Here's how the part is built. I have some questions about the finished solid (model axes, mm). Round coordinates to 2 decimals unless told otherwise and drop trailing zeros. Order: outer loops, then holes, each group sorted by start corner. A loop starts at its lowest first (then second) coordinate and runs counter-clockwise, first axis right, second up.
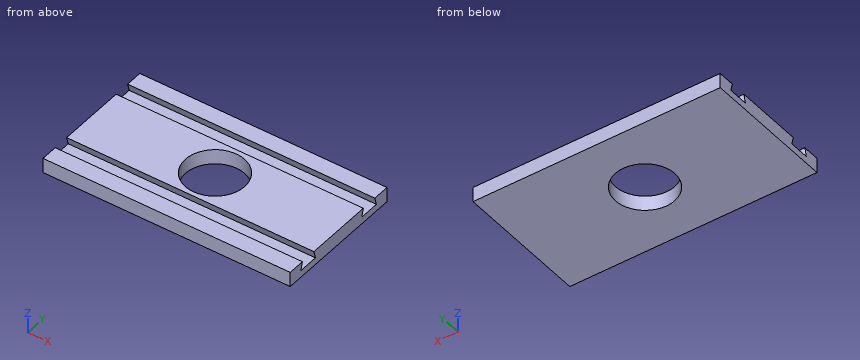
```python
from build123d import *

# Parameters (mm, degrees)
PLATE_PROFILE_W             = 100
PLATE_PROFILE_H             = 54
PLATE_PROFILE_R             = 12
PLATE_6MM_DEPTH             = 6
DOVETAIL_GROOVES_DEPTH      = 58.140178509
DOVETAIL_GROOVES_DEPTH_BACK = 58.140178509


with BuildPart() as part:
    # Plate profile → Plate 6mm (new body)
    with BuildSketch(Plane.XY):
        Rectangle(PLATE_PROFILE_W, PLATE_PROFILE_H)
        Circle(PLATE_PROFILE_R, mode=Mode.SUBTRACT)
    extrude(amount=-PLATE_6MM_DEPTH)

    # Groove profiles → Dovetail grooves (cut, two sides: drawn at the far end of the back side and taken through both)
    with BuildSketch(Plane(origin=(0, 0, 0), x_dir=(0, 0, -1), z_dir=(1, 0, 0)).offset(-DOVETAIL_GROOVES_DEPTH_BACK)):
        Polygon((-0.2, 13.846344337), (3.2, 12.939677671), (3.2, 21.060322329), (-0.2, 20.153655663), align=None)
        Polygon((-0.2, -13.846344337), (3.2, -12.939677671), (3.2, -21.060322329), (-0.2, -20.153655663), align=None)
    extrude(amount=DOVETAIL_GROOVES_DEPTH + DOVETAIL_GROOVES_DEPTH_BACK, mode=Mode.SUBTRACT)


solid = part.part
```
1) If we section it at A-A (y = 0): Write out the boundary of the cut face in (x, z), plus the area to 3 significant figures.
2) I'm going to push flat-ended pins straight in: pin 1 (6.5 mm diameter, centred on x = 9.5, y = -17, fed in from +Z); pin 2 (4 mm diameter, centred on x = 0, y = 16, fed in from +Z). Where does each tip first touch, or does it pass through?
3) If we section it at D-D (z = -4.7): Write out the boundary of the cut face in (x, y), plus the area to 3 significant figures.
4) If we section it at B-B (x = 0): Write out the boundary of the cut face in (y, z), plus the area to 3 significant figures.
5) If we section it at C-C (x = 23.5): Write out the boundary of the cut face in (y, z).
6) I need wall thicknesses on line 1 (Y direction, x = -42, z = -2.2); line 2 (Y direction, x = 0, z = -4.4); line 3 (Z direction, x = -32, y = 19). Which ranges of each line are inside material? Lowest first, please.
Solutions:
1. outline: (-50, -6) - (-12, -6) - (-12, 0) - (-50, 0) - close; (12, -6) - (50, -6) - (50, 0) - (12, 0) - close
1. area: 456 mm2
2. pin 1: stops at z = 0
2. pin 2: stops at z = -3.2
3. outline: (-50, -27) - (50, -27) - (50, 27) - (-50, 27) - close; hole circle Ø24 at (0, 0)
3. area: 4,950 mm2
4. outline: (-27, -6) - (-12, -6) - (-12, 0) - (-13.79, 0) - (-12.94, -3.2) - (-21.06, -3.2) - (-20.21, 0) - (-27, 0) - close; (12, -6) - (27, -6) - (27, 0) - (20.21, 0) - (21.06, -3.2) - (12.94, -3.2) - (13.79, 0) - (12, 0) - close
4. area: 133 mm2
5. outline: (-27, -6) - (27, -6) - (27, 0) - (20.21, 0) - (21.06, -3.2) - (12.94, -3.2) - (13.79, 0) - (-13.79, 0) - (-12.94, -3.2) - (-21.06, -3.2) - (-20.21, 0) - (-27, 0) - close
6. line 1: y = -27 to -20.79, -13.21 to 13.21, 20.79 to 27
6. line 2: y = -27 to -12, 12 to 27
6. line 3: z = -6 to -3.2
